Geometry check sheet. Reference: the model listing, model coordinates, mm. A direction names the side the tool comes from. Give positions to 0.01 mm unless a question says otherwise; leave off trailing zeros. Loops run counter-clockwise (first coordinate to the right, second up) from the corner with the lowest first, then second, coordinate; pieces in that order, holes last. Notation, with made-up numbers: (6.5, -11.75) -> (48.5, -11.75) arc R9 cw to (48.5, 4.25) -> close; hole circle Ø4 at (73, 0.5). An arc over 180 degrees is marked (long way). Answer in a Markdown table with one row per item. Add a question column.
```python
from build123d import *

# Parameters (mm, degrees)
ESQUISSE1_W        = 431
ESQUISSE1_H        = 560
ESQUISSE1_W_2      = 331
ESQUISSE1_H_2      = 200
BOSS_EXTRU_1_DEPTH = 24
BOSS_EXTRU_2_DEPTH = 15


with BuildPart() as part:
    # Esquisse1 → Boss.-Extru.1 (new body)
    with BuildSketch(Plane(origin=(0, 0, 0), x_dir=(1, 0, 0), z_dir=(0, 1, 0))):
        Rectangle(ESQUISSE1_W, ESQUISSE1_H)
        with Locations((0, 130)):
            Rectangle(ESQUISSE1_W_2, ESQUISSE1_H_2, mode=Mode.SUBTRACT)
    extrude(amount=BOSS_EXTRU_1_DEPTH)

    # Esquisse2 → Boss.-Extru.2 (add)
    with BuildSketch(Plane(origin=(0, 24, 0), x_dir=(1, 0, 0), z_dir=(0, 1, 0))):
        Polygon((-215.5, 280), (215.5, 280), (215.5, -280), (191.5, -280), (191.5, 256), (-191.5, 256), (-191.5, -280), (-215.5, -280), align=None)
    extrude(amount=BOSS_EXTRU_2_DEPTH)


solid = part.part
```
1. Release check for a two-part mould opening along Z. For faces 1 (the face through (-165.5, 12, -129)), 2 (the face through (165.5, 12, -129)), 3 (the face through (191.5, 31, 16)), 4 (the face through (-3, 19, -280)) record: released by +Z, released by -Z, zero draft, split by the parting line, or undercut.
2. Sectioned sample at C-C (y = 12.5). Enter the section's corners in (x, z).
3. Sectioned sample at D-D (z = 41.5). Enter the section's corners in (x, y), plus the area to 3 significant figures.
4. Access from +Z, -Z, +X, -X, +Y, -Y to the whole of each face (thin tool, end or side, straight path). Record for faces 5 (the face through (-2, 12, -30)), 6 (the face through (-191.5, 31, 8)), 7 (the face through (215.5, 19, -4)).
5. Sectioned sample at B-B (z = -155.5). Enter the section's corners in (x, y), plus the area to 3 significant figures.
6. Gauge pin test, flat ends, axial feed: pin 1 Ø1.5 at (x, y) = (-56.5, 28.5) entering from +Z; pin 2 Ø6 at (x, z) = (129, 152.5) entering from +Y. Record the tip position at first contact, or that the pin passes through.
7. Material ranges on L1, parallel to X at y = 27, z = 228.5; L2, parallel to Z at x = -85, y = 14.5; L3, parallel to Y at x = 128, z = 89, recorded low to high. Write a range as from..to.
8. Sectioned sample at A-A (x = -19.5). Enter the section's corners in (y, z), plus the area to 3 significant figures.
Response:
| question | item | result |
|---|---|---|
| 1 | face 1 | undercut |
| 1 | face 2 | undercut |
| 1 | face 3 | zero draft |
| 1 | face 4 | released by -Z |
| 2 | outline | (-215.5, -280) -> (215.5, -280) -> (215.5, 280) -> (-215.5, 280) -> close; hole (-165.5, -230) -> (165.5, -230) -> (165.5, -30) -> (-165.5, -30) -> close |
| 3 | outline | (-215.5, 0) -> (215.5, 0) -> (215.5, 39) -> (191.5, 39) -> (191.5, 24) -> (-191.5, 24) -> (-191.5, 39) -> (-215.5, 39) -> close |
| 3 | area | 11,100 mm2 |
| 4 | face 5 | +Y, -Y |
| 4 | face 6 | +Z, +Y |
| 4 | face 7 | +Z, -Z, +X, +Y, -Y |
| 5 | outline | (-215.5, 0) -> (-165.5, 0) -> (-165.5, 24) -> (-191.5, 24) -> (-191.5, 39) -> (-215.5, 39) -> close; (165.5, 0) -> (215.5, 0) -> (215.5, 39) -> (191.5, 39) -> (191.5, 24) -> (165.5, 24) -> close |
| 5 | area | 3,120 mm2 |
| 6 | pin 1 | stops at z = -256 |
| 6 | pin 2 | stops at y = 24 |
| 7 | L1 | x = -215.5..-191.5, 191.5..215.5 |
| 7 | L2 | z = -280..-230, -30..280 |
| 7 | L3 | y = 0..24 |
| 8 | outline | (0, -280) -> (39, -280) -> (39, -256) -> (24, -256) -> (24, -230) -> (0, -230) -> close; (0, -30) -> (24, -30) -> (24, 280) -> (0, 280) -> close |
| 8 | area | 9,000 mm2 |
